Autodesk Inventor part; units mm, degrees
ref_plane "YZ Plane" through (0, 0, 0) normal (1, 0, 0) x (0, 1, 0)
ref_plane "XZ Plane" through (0, 0, 0) normal (0, 1, 0) x (-1, 0, 0)
ref_plane "XY Plane" through (0, 0, 0) normal (0, 0, 1) x (1, 0, 0)
sketch "Sketch1" plane through (0, 0, 0) normal (0, 1, 0) x (-1, 0, 0)
  line L0 (0, 0) -> (100, 0)
  line L1 (100, 0) -> (100, -200)
  line L2 (100, -200) -> (0, -200)
  line L3 (0, -200) -> (0, 0)
  line L4 (82, -67.5) -> (18, -67.5)
  line L5 (18, -67.5) -> (18, -132.5)
  line L6 (18, -132.5) -> (82, -132.5)
  line L7 (82, -132.5) -> (82, -67.5)
  point P0 (100, -100)
  dimension "d0" = 200
  dimension "d1" = 100
  dimension "d2" = 65
  dimension "d3" = 64
  dimension "d4" = 18
  dimension "d5" = 67.5
extrude "Extrusion1" add sketch "Sketch1" along normal blind 3
properties part number "Q top1 new" material "ABS Plastic"
Verification items for the finished model (mm, model axes). Coordinates: 2 decimals unless noted, no trailing zeros. Order: outer loops, then holes, each group sorted by start corner. A loop starts at its lowest first (then second) coordinate and runs counter-clockwise, first axis right, second up. Notation, with made-up numbers: (72, -10) -> (79, -10) arc R9 cw to (79, -5) -> close; hole circle Ø3 at (85.5, -27). An arc over 180 degrees is marked (long way). Use CSV: the item, a comma, the result in double quotes. Start each with the question number.
Q1. Section check C-C, the plane y = 2.25. Record the cut outline in (x, z).
Q2. Thickness scan on line 1 along X through (y, z) = (1.7, -71.5); line 2 along Z through (x, y) = (-44.5, 2.8). Record the ranges inside material, lowest first.
Q3. Section check B-B, the plane x = -76.5. Record the cut outline in (y, z), and give its area (3 significant figures).
Q4. Section check A-A, the plane z = -112. Record the cut outline in (x, y).
Returned:
1,outline,"(-100, -200) -> (0, -200) -> (0, 0) -> (-100, 0) -> close; hole (-82, -132.5) -> (-18, -132.5) -> (-18, -67.5) -> (-82, -67.5) -> close"
2,line 1,"x = -100 to -82, -18 to 0"
2,line 2,"z = -200 to -132.5, -67.5 to 0"
3,outline,"(0, -200) -> (3, -200) -> (3, -132.5) -> (0, -132.5) -> close; (0, -67.5) -> (3, -67.5) -> (3, 0) -> (0, 0) -> close"
3,area,"405 mm^2"
4,outline,"(-100, 0) -> (-82, 0) -> (-82, 3) -> (-100, 3) -> close; (-18, 0) -> (0, 0) -> (0, 3) -> (-18, 3) -> close"
